The listing builds one solid part. Answer for the finished solid, in the listing's coordinates (mm). Give positions to 0.01 mm unless a question says otherwise; leave off trailing zeros. Order: outer loops, then holes, each group sorted by start corner. A loop starts at its lowest first (then second) coordinate and runs counter-clockwise, first axis right, second up. Notation, with made-up numbers: (85.25, -5) - (97.25, -5) arc R28 ccw to (97.25, 29) - close; hole circle Ø11 at (32, 75). An arc over 180 degrees is marked (long way). Answer in a Markdown table with one row per item. Add a question column.
```python
from build123d import *

# Parameters (mm, degrees)
F0_W     = 25
F0_H     = 25
F1_DEPTH = 4
F2_D     = 3


# Not quite as in the source:
# - a feature names something its author has since deleted; it is built from what else it names


with BuildPart() as f1:
    # F0 (on Top) → F1 (new body)
    with BuildSketch(Plane.XY):
        Rectangle(F0_W, F0_H)
    extrude(amount=F1_DEPTH)

    # F2 (through all)
    with Locations(Plane(origin=(0, 0, 0), x_dir=(1, 0, 0), z_dir=(0, 0, -1))):
        with Locations((-7.5, 0), (7.5, 0), (0, -7), (0, 7)):
            Hole(F2_D / 2)


solid = f1.part
```
(1) Find section A-A, the plane y = 0. Write down the section's boundary in (x, z), plus the area to 3 significant figures.
(2) Find section C-C, the plane z = 2.8. Write down the section's boundary in (x, y).
(3) Straight lines are drawn through the part: line 1 (Y direction, x = 0, z = 2.3); line 2 (X direction, y = -7, z = 0.9). For each, find the intervals that lie inside material, in ascending order.
(4) The mould has two halves that part along X. Classify faces 1 (the face through (-6, 0, 2)), 2 (the face through (-12.5, 0, 2)), 3 (the face through (9, 0, 2)), 4 (the face through (12.5, 0, 2)): +X half, -X half, draft (parallel to the pull), parting line (faces both ways), or undercut.
(5) Find section B-B, the plane x = 0. Write down the section's boundary in (y, z).
(6) Find section D-D, the plane y = 7. Write down the section's boundary in (x, z).
Answer key:
| question | item | result |
|---|---|---|
| 1 | outline | (-12.5, 0) - (-9, 0) - (-9, 4) - (-12.5, 4) - close; (-6, 0) - (6, 0) - (6, 4) - (-6, 4) - close; (9, 0) - (12.5, 0) - (12.5, 4) - (9, 4) - close |
| 1 | area | 76.0 mm² |
| 2 | outline | (-12.5, -12.5) - (12.5, -12.5) - (12.5, 12.5) - (-12.5, 12.5) - close; hole circle Ø3 at (-7.5, 0); hole circle Ø3 at (0, -7); hole circle Ø3 at (0, 7); hole circle Ø3 at (7.5, 0) |
| 3 | line 1 | -12.5 to -8.5, -5.5 to 5.5, 8.5 to 12.5 |
| 3 | line 2 | -12.5 to -1.5, 1.5 to 12.5 |
| 4 | face 1 | undercut |
| 4 | face 2 | -X half |
| 4 | face 3 | undercut |
| 4 | face 4 | +X half |
| 5 | outline | (-12.5, 0) - (-8.5, 0) - (-8.5, 4) - (-12.5, 4) - close; (-5.5, 0) - (5.5, 0) - (5.5, 4) - (-5.5, 4) - close; (8.5, 0) - (12.5, 0) - (12.5, 4) - (8.5, 4) - close |
| 6 | outline | (-12.5, 0) - (-1.5, 0) - (-1.5, 4) - (-12.5, 4) - close; (1.5, 0) - (12.5, 0) - (12.5, 4) - (1.5, 4) - close |
